Verification items for the finished model (mm, model axes). A direction names the side the tool comes from. Coordinates: 2 decimals unless noted, no trailing zeros. Order: outer loops, then holes, each group sorted by start corner. A loop starts at its lowest first (then second) coordinate and runs counter-clockwise, first axis right, second up. Notation, with made-up numbers: (33.5, 64.25) - (71.5, 64.25) arc R28 cw to (71.5, 85.25) - close; hole circle Ø4 at (-25.75, 14). An arc over 180 degrees is marked (long way). Answer as CSV lines item,"result". Start each with the question number.
1. Set-up check for faces 1 (the flat face through (-30, 34, 49)), 2 (the cylindrical face through (30.18, 37.53, 52.39)), 3 (the flat face through (-32.902, -3.401, 50.507)): record each of +Z, -Z, +X, -X, +Y, -Y from which the full face is reachable in a straight line by a thin tool's end or side.
2. Mould release check, pull along Z, two halves, no side actions. Record for faces 4 (the flat face through (3, -11, 52)), 5 (the flat face through (30, 35, 51)), 6 (the cylindrical face through (30.1, 37, 47.5)): pulls with the +Z half, pulls with the -Z half, needs draft (parallel to the pull), parting line crosses it, or undercut.
3. Section check D-D (y = 7.5). Record the cut outline in (x, z).
4. Material ranges on L1, parallel to Y at x = 25.5, z = 51.7; L2, parallel to Z at x = -30, y = 38.5; L3, parallel to X at y = 23, z = 51.2, recorded low to high. Write a range as [from, to].
5. Go/stop test with flat-tipped pins: pin 1 (3.5 mm diameter, centred on x = 25.5, y = 25.5, fed in from -Z); pin 2 (15 mm diameter, centred on x = 16, y = 5.5, fed in from -Z). Record where each tip stops, or that it passes through.
6. Section check A-A (x = 10). Record the cut outline in (y, z).
7. Section check B-B (x = 25.5). Record the cut outline in (y, z), and give its area (3 significant figures).
8. Section check C-C (y = -4.5). Record the cut outline in (x, z).
from build123d import *

# Parameters (mm, degrees)
SKETCH003_R     = 11.5
SKETCH003_R_2   = 2
SKETCH003_R_3   = 4.75
SKETCH003_W     = 14
SKETCH003_H     = 5
PAD001_DEPTH    = 5
PAD013_DEPTH    = 6
SKETCH048_R     = 1.4
POCKET038_DEPTH = 5
CHAMFER019_SIZE = 1
CHAMFER020_SIZE = 1
CHAMFER021_SIZE = 1
FILLET_R        = 2


with BuildPart() as part:
    # Sketch003 → Pad001 (new body)
    with BuildSketch(Plane.XY):
        Polygon((-40, 40), (40, 40), (40, -3), (32, -11), (-26, -11), (-40, 3), align=None)
        with Locations((10, 10)):
            Circle(SKETCH003_R, mode=Mode.SUBTRACT)
        with Locations((-35, 12)):
            Circle(SKETCH003_R_2, mode=Mode.SUBTRACT)
        with Locations((35, 12)):
            Circle(SKETCH003_R_2, mode=Mode.SUBTRACT)
        with Locations((25.5, -5.5)):
            Circle(SKETCH003_R_2, mode=Mode.SUBTRACT)
        with Locations((-5.5, 25.5)):
            Circle(SKETCH003_R_2, mode=Mode.SUBTRACT)
        with Locations((-31, 23)):
            Circle(SKETCH003_R_3, mode=Mode.SUBTRACT)
        with Locations((25.5, 25.5)):
            Circle(SKETCH003_R_2, mode=Mode.SUBTRACT)
        with Locations((-5.5, -5.5)):
            Circle(SKETCH003_R_2, mode=Mode.SUBTRACT)
        with Locations((-4.017783, 33.539897)):
            Rectangle(SKETCH003_W, SKETCH003_H, mode=Mode.SUBTRACT)
    extrude(amount=PAD001_DEPTH)

    # Sketch047 → Pad013 (join)
    with BuildSketch(Plane(origin=(0, 40, 0), x_dir=(-1, 0, 0), z_dir=(0, 1, 0))):
        with BuildLine():
            ThreePointArc((-33.5, 1.000024), (-30, -2.5), (-26.5, 1.000024))
            Line((-33.5, 1.000024), (-26.5, 1.000024))
        make_face()
        with BuildLine():
            ThreePointArc((26.5, 1.000024), (30, -2.5), (33.5, 1.000024))
            Line((26.5, 1.000024), (33.5, 1.000024))
        make_face()
    extrude(amount=-PAD013_DEPTH)

    # Sketch048 → Pocket038 (cut)
    with BuildSketch(Plane(origin=(0, 40, 0), x_dir=(-1, 0, 0), z_dir=(0, 1, 0))):
        with Locations((-30, 1)):
            Circle(SKETCH048_R)
        with Locations((30, 1)):
            Circle(SKETCH048_R)
    extrude(amount=-POCKET038_DEPTH, mode=Mode.SUBTRACT)

    # Chamfer019
    chamfer019_edges = [part.edges().sort_by_distance(p)[0] for p in [
        (40, 18.5, 5),
        (-40, 21.5, 5),
        (-33, -4, 5),
        (3, -11, 5),
        (36, -7, 5),
    ]]
    chamfer(chamfer019_edges, length=CHAMFER019_SIZE)

    # Chamfer020
    chamfer020_edges = [part.edges().sort_by_distance(p)[0] for p in [
        (36, -7, 0),
        (3, -11, 0),
        (-33, -4, 0),
    ]]
    chamfer(chamfer020_edges, length=CHAMFER020_SIZE)

    # Chamfer021
    chamfer021_edges = [part.edges().sort_by_distance(p)[0] for p in [
        (-35.75, 23, 5),
    ]]
    chamfer(chamfer021_edges, length=CHAMFER021_SIZE)

    # Fillet
    fillet_edges = [part.edges().sort_by_distance(p)[0] for p in [
        (-35.75, 23, 4),
    ]]
    fillet(fillet_edges, radius=FILLET_R)


with BuildPart() as part_1:
    # Body001 placement: moved
    add(part.part.moved(Location((0, 0, 50))))


solid = part_1.part
Evaluation:
1,face 1,"-Z, +X, -X, -Y"
1,face 2,"+Y"
1,face 3,"-Z, -X, -Y"
2,face 4,"needs draft"
2,face 5,"undercut"
2,face 6,"pulls with the -Z half"
3,outline,"(-40, 50) - (-1.22, 50) - (-1.22, 55) - (-39, 55) - (-40, 54) - close; (21.22, 50) - (40, 50) - (40, 54) - (39, 55) - (21.22, 55) - close"
4,L1,"y = [-11, -7.5], [-3.5, 23.5], [27.5, 40]"
4,L2,"z = [47.5, 49.6], [52.4, 55]"
4,L3,"x = [-40, -35.75], [-26.25, 40]"
5,pin 1,"passes through"
5,pin 2,"stops at z = 50"
6,outline,"(-11, 51) - (-10, 50) - (-1.5, 50) - (-1.5, 55) - (-10, 55) - (-11, 54) - close; (21.5, 50) - (40, 50) - (40, 55) - (21.5, 55) - close"
7,outline,"(-11, 51) - (-10, 50) - (-7.5, 50) - (-7.5, 55) - (-10, 55) - (-11, 54) - close; (-3.5, 50) - (23.5, 50) - (23.5, 55) - (-3.5, 55) - close; (27.5, 50) - (40, 50) - (40, 55) - (27.5, 55) - close"
7,area,"214 mm²"
8,outline,"(-32.5, 51) - (-31.09, 50) - (-7.23, 50) - (-7.23, 55) - (-31.09, 55) - (-32.5, 54) - close; (-3.77, 50) - (23.77, 50) - (23.77, 55) - (-3.77, 55) - close; (27.23, 50) - (37.09, 50) - (38.5, 51) - (38.5, 54) - (37.09, 55) - (27.23, 55) - close"
